from build123d import *

# Parameters (mm, degrees)
ESTRUSIONE_ESTRUSIONE1_DEPTH = 3.75
RACCORDO2_R                  = 1
SCHIZZO3_R                   = 1.75
TAGLIO_ESTRUSIONE1_DEPTH     = 10


with BuildPart() as part:
    # Schizzo1 → Estrusione-Estrusione1 (new body, symmetric)
    with BuildSketch(Plane(origin=(0, 0, 0), x_dir=(0, 0, -1), z_dir=(1, 0, 0))):
        with BuildLine():
            Line((-30, 22), (-30, 21))
            ThreePointArc((-30, 21), (-25, 16), (-30, 11))
            Line((-30, 11), (-30, 10))
            ThreePointArc((-30, 10), (-29.075946517, 10.07158325), (-28.173941951, 10.284624946))
            Line((-28.173941951, 10.284624946), (-14.279791844, 1.720208156))
            ThreePointArc((-14.279791844, 1.720208156), (-15.496162696, 1.216370852), (-16, 0))
            Line((-16, 0), (16, 0))
            ThreePointArc((16, 0), (15.496162696, 1.216370852), (14.279791844, 1.720208156))
            Line((14.279791844, 1.720208156), (28.173941951, 10.284624946))
            ThreePointArc((28.173941951, 10.284624946), (29.075946517, 10.07158325), (30, 10))
            Line((30, 10), (30, 11))
            ThreePointArc((30, 11), (25, 16), (30, 21))
            Line((30, 21), (30, 22))
            ThreePointArc((30, 22), (28.020680207, 21.664123335), (26.262962858, 20.694097719))
            Line((26.262962858, 20.694097719), (4, 2.970240215))
            Line((4, 2.970240215), (-4, 2.970240215))
            Line((-4, 2.970240215), (-26.262962858, 20.694097719))
            ThreePointArc((-26.262962858, 20.694097719), (-28.020680207, 21.664123335), (-30, 22))
        make_face()
        with BuildLine():
            Line((-20.125796974, 10.754754637), (-12.80100478, 5.593685162))
            ThreePointArc((-12.80100478, 5.593685162), (-12.653117343, 4.740293889), (-13.506508616, 4.592406452))
            Line((-13.506508616, 4.592406452), (-20.83130081, 9.753475926))
            ThreePointArc((-20.83130081, 9.753475926), (-20.979188247, 10.606867199), (-20.125796974, 10.754754637))
        make_face(mode=Mode.SUBTRACT)
        with BuildLine():
            Line((20.125796974, 10.754754637), (12.80100478, 5.593685162))
            ThreePointArc((12.80100478, 5.593685162), (12.653117343, 4.740293889), (13.506508616, 4.592406452))
            Line((13.506508616, 4.592406452), (20.83130081, 9.753475926))
            ThreePointArc((20.83130081, 9.753475926), (20.979188247, 10.606867199), (20.125796974, 10.754754637))
        make_face(mode=Mode.SUBTRACT)
    extrude(amount=ESTRUSIONE_ESTRUSIONE1_DEPTH, both=True)

    # Raccordo2
    raccordo2_edges = [part.edges().sort_by_distance(p)[0] for p in [
        (0, 2.970240215, 4),
        (0, 2.970240215, -4),
        (0, 10.284624946, -28.173941951),
        (0, 1.720208156, -14.279791844),
        (0, 1.720208156, 14.279791844),
        (0, 10.284624946, 28.173941951),
    ]]
    fillet(raccordo2_edges, radius=RACCORDO2_R)

    # Schizzo3 → Taglio-Estrusione1 (cut)
    with BuildSketch(Plane.XZ):
        with Locations((0, 12)):
            Circle(SCHIZZO3_R)
    taglio_estrusione1 = extrude(amount=-TAGLIO_ESTRUSIONE1_DEPTH, mode=Mode.SUBTRACT)

    # Specchia1: Taglio-Estrusione1 across plane
    add(taglio_estrusione1.mirror(Plane.XY), mode=Mode.SUBTRACT)


solid = part.part
Geometry: final body of the model. Coordinates: model frame, mm. A direction names the side the tool comes from. Coordinates: 2 decimals unless noted, no trailing zeros. Order: outer loops, then holes, each group sorted by start corner. A loop starts at its lowest first (then second) coordinate and runs counter-clockwise, first axis right, second up.
(1) Section query A-A (y = 16). Return the cut outline in (x, z).
(2) Section query B-B (z = 12). Return the cut outline in (x, y).
(3) Draft query along Y for faces 1 (the face through (0.1, 10.5, 30)), 2 (the face through (0.1, 8.2, -16.5)), 3 (the face through (0.053, 21.655, 27.994)), 4 (the face through (0, 16, 25)). Return one class per face: pulls with the +Y half, pulls with the -Y half, needs draft (parallel to the pull), parting line crosses it, or undercut.
(4) First-contact query: pin 1 (0.5 mm diameter, centred on x = 0, z = 13, fed in from -Y); pin 2 (2 mm diameter, centred on x = 0.5, z = 2, fed in from +Y); pin 3 (4 mm diameter, centred on x = 1, y = 16, fed in from -Z). Flat tips, straight axial feed; report the tip coordinate or a pass-through.
(5) Section query C-C (x = 0). State how many separate pieces and enclosed holes the cut face has, plus the area to 3 significant figures.
(6) Access query for faces 5 (the face through (0.053, 10.043, 29.287)), 6 (the face through (0.05, 12.06, -15.42)), 7 (the face through (0.053, 1.936, 15.327)), 8 (the face through (0.05, 7.14, -17.12)). Directions: +Z, -Z, +X, -X, +Y, -Y. A direction counts if a zero-diameter tool reaches every point of the face in a straight line with its end or side. Return the directions, or none.
(7) Section query D-D (z = 22.5). Return the cut outline in (x, y), plus the area to 3 significant figures.
(8) Material intervals for probe 1 along X at (y, z) = (3.75, 12); probe 2 along Z at (x, y) = (3, 10.25); probe 3 along Z at (x, y) = (0, 2.5), sorted ascending.
Solution:
1. outline: (-3.75, -25) - (3.75, -25) - (3.75, -20.37) - (-3.75, -20.37) - close; (-3.75, 20.37) - (3.75, 20.37) - (3.75, 25) - (-3.75, 25) - close
2. outline: (-3.75, 0) - (-1.75, 0) - (-1.75, 9.34) - (-3.75, 9.34) - close; (1.75, 0) - (3.75, 0) - (3.75, 9.34) - (1.75, 9.34) - close
3. face 1: needs draft
3. face 2: undercut
3. face 3: pulls with the +Y half
3. face 4: undercut
4. pin 1: stops at y = 10
4. pin 2: stops at y = 2.97
4. pin 3: stops at z = -25.42
5. separate pieces: 3
5. enclosed holes: 0
5. area: 349 mm2
6. face 5: +X, -X, -Y
6. face 6: +X, -X, +Y
6. face 7: +Z, +X, -X
6. face 8: +X, -X
7. outline: (-3.75, 6.79) - (3.75, 6.79) - (3.75, 17.7) - (-3.75, 17.7) - close
7. area: 81.8 mm2
8. probe 1: x = -3.75 to -1.75, 1.75 to 3.75
8. probe 2: z = -30 to -21.09, -19.41 to -13.14, 13.14 to 19.41, 21.09 to 30
8. probe 3: z = -15.6 to -13.75, -10.25 to 10.25, 13.75 to 15.6
